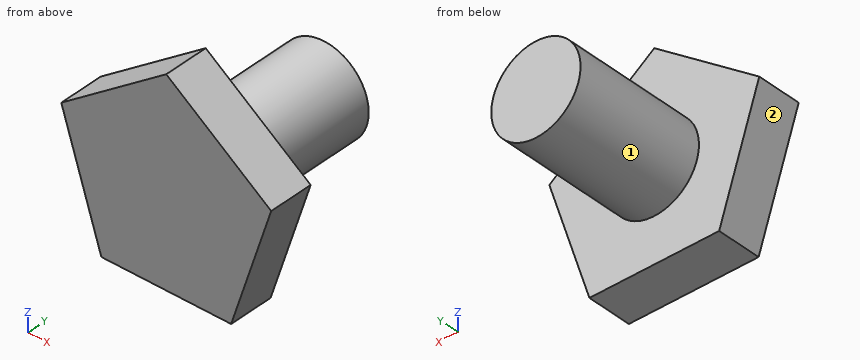
```python
from build123d import *

# Parameters (mm, degrees)
F0_R     = 25.4
F1_DEPTH = 76.2
F3_DEPTH = 25.4


with BuildPart() as f1:
    # F0 (on Front) → F1 (new body)
    with BuildSketch(Plane.XZ):
        Circle(F0_R)
    extrude(amount=F1_DEPTH)

    # F2 (on face) → F3 (join)
    with BuildSketch(Plane.XZ.offset(76.2)):
        Polygon((36.90836, -50.8), (59.718982, 19.403873), (0, 62.792253), (-59.718982, 19.403873), (-36.90836, -50.8), align=None)
    extrude(amount=F3_DEPTH)


solid = f1.part
```
Geometry check sheet. Reference: the model listing, model coordinates, mm. Face numbers are marked on the shaded views. A direction names the side the tool comes from. Round coordinates to 2 decimals unless told otherwise and drop trailing zeros. Loops run counter-clockwise (first coordinate to the right, second up) from the corner with the lowest first, then second, coordinate; pieces in that order, holes last. Notation, with made-up numbers: (-29, -27) - (9, -27) arc R11 ccw to (9, -9) - close; hole circle Ø8 at (-30.5, 2). An arc over 180 degrees is marked (long way). Write each question's results on one line, items separated by ' | '. Start each with the question number.
Q1. Cross-section at D-D on z = 22.5. Enter the section's corners in (x, y).
Q2. Gauge pin test, flat ends, axial feed: P1, Ø10, axis at x = 33.5, z = 13.5, coming from the +Y side; P2, Ø10, axis at x = -13.5, y = -22, coming from the -Z side; P3, Ø10, axis at y = -91, z = 2.5, coming from the -X side. Record the tip position at first contact, or that the pin passes through.
Q3. Access from +Z, -Z, +X, -X, +Y, -Y to the whole of each face (thin tool, end or side, straight path). Record for the marked faces 1 and 2.
Q4. Cross-section at A-A on y = -24.5. Enter the section's corners in (x, z), and give its area (3 significant figures).
Q5. Cross-section at B-B on z = 2.5. Enter the section's corners in (x, y).
Q6. Cross-section at C-C on x = 50. Enter the section's corners in (y, z).
Q7. Thickness scan on line 1 (Y direction, x = -19, z = 38); line 2 (Z direction, x = 0, y = -60.5); line 3 (X direction, y = -72.5, z = -1). Record the ranges inside material, lowest first. Write a range as [from, to].
Answers below:
1) outline: (-55.46, -101.6) - (55.46, -101.6) - (55.46, -76.2) - (11.79, -76.2) - (11.79, 0) - (-11.79, 0) - (-11.79, -76.2) - (-55.46, -76.2) - close
2) P1: stops at y = -76.2 | P2: stops at z = -23.94 | P3: stops at x = -55.85
3) face 1: +Y | face 2: -Z, -X, +Y, -Y
4) outline: circle Ø50.8 at (0, 0) | area: 2,030 mm²
5) outline: (-54.23, -101.6) - (54.23, -101.6) - (54.23, -76.2) - (25.28, -76.2) - (25.28, 0) - (-25.28, 0) - (-25.28, -76.2) - (-54.23, -76.2) - close
6) outline: (-101.6, -10.51) - (-76.2, -10.51) - (-76.2, 26.47) - (-101.6, 26.47) - close
7) line 1: y = [-101.6, -76.2] | line 2: z = [-25.4, 25.4] | line 3: x = [-25.38, 25.38]
